```python
from build123d import *

# Parameters (mm, degrees)
F0_R     = 11.2
F1_DEPTH = 7


with BuildPart() as f1:
    # F0 (on Top) → F1 (new body)
    with BuildSketch(Plane.XY):
        with BuildLine():
            ThreePointArc((-0.9650827881, 13.1646730006), (-8.6022624346, 10.012046794), (-12.8691579618, 2.9367964443))
            ThreePointArc((-12.8691579618, 2.9367964443), (-13.1863620091, 0.599880793), (-13.0826534178, -1.7561832335))
            ThreePointArc((-13.0826534178, -1.7561832335), (-8.9594650145, -9.693708612), (-0.722399634, -13.1802177057))
            ThreePointArc((-0.722399634, -13.1802177057), (0, -13.1604354113), (0.722399634, -13.1802177057))
            ThreePointArc((0.722399634, -13.1802177057), (8.0432942537, -10.4663946777), (12.5501283831, -4.0907551342))
            ThreePointArc((12.5501283831, -4.0907551342), (13.0365197552, -2.0710269606), (13.2, 0))
            ThreePointArc((13.2, 0), (9.6689992451, 8.9861256167), (0.9650827881, 13.1646730006))
            ThreePointArc((0.9650827881, 13.1646730006), (0, 13.1293460011), (-0.9650827881, 13.1646730006))
        make_face()
        Circle(F0_R, mode=Mode.SUBTRACT)
        with BuildLine():
            ThreePointArc((-13.0826534178, -1.7561832335), (-13.1863620091, 0.599880793), (-12.8691579618, 2.9367964443))
            ThreePointArc((-12.8691579618, 2.9367964443), (-18.9175577348, 12.787783411), (-12.6283316175, 22.4867894878))
            ThreePointArc((-12.6283316175, 22.4867894878), (-13.0313646183, 24.2261255691), (-13.1959884441, 26.0039401262))
            ThreePointArc((-13.1959884441, 26.0039401262), (-24.637001113, 12.0769373767), (-13.0826534178, -1.7561832335))
        make_face()
        with BuildLine():
            ThreePointArc((-12.6283316175, 22.4867894878), (-8.2414011401, 16.0182205898), (-0.9650827881, 13.1646730006))
            ThreePointArc((-0.9650827881, 13.1646730006), (0, 13.2), (0.9650827881, 13.1646730006))
            ThreePointArc((0.9650827881, 13.1646730006), (9.6689992451, 17.3432203845), (13.2, 26.3293460011))
            ThreePointArc((13.2, 26.3293460011), (-0.1627153004, 39.5283430741), (-13.1959884441, 26.0039401262))
            ThreePointArc((-13.1959884441, 26.0039401262), (-13.0313646183, 24.2261255691), (-12.6283316175, 22.4867894878))
        make_face()
        with Locations((0, 26.3293460011)):
            Circle(F0_R, mode=Mode.SUBTRACT)
        with BuildLine():
            ThreePointArc((0.9650827881, 13.1646730006), (0, 13.2), (-0.9650827881, 13.1646730006))
            ThreePointArc((-0.9650827881, 13.1646730006), (0, 13.1293460011), (0.9650827881, 13.1646730006))
        make_face()
        with BuildLine():
            ThreePointArc((0.722399634, -13.1802177057), (0, -13.1604354113), (-0.722399634, -13.1802177057))
            ThreePointArc((-0.722399634, -13.1802177057), (0, -13.2), (0.722399634, -13.1802177057))
        make_face()
        with BuildLine():
            ThreePointArc((0.722399634, -13.1802177057), (0, -13.2), (-0.722399634, -13.1802177057))
            ThreePointArc((-0.722399634, -13.1802177057), (-10.4506279527, -34.4242047158), (12.566049408, -30.4020195408))
            ThreePointArc((12.566049408, -30.4020195408), (13.0405493018, -28.4059363053), (13.2, -26.3604354113))
            ThreePointArc((13.2, -26.3604354113), (13.1998442738, -26.2963171862), (13.199377099, -26.2322004739))
            ThreePointArc((13.199377099, -26.2322004739), (9.5416209523, -17.2391707181), (0.722399634, -13.1802177057))
        make_face()
        with Locations((0, -26.3604354113)):
            Circle(F0_R, mode=Mode.SUBTRACT)
        with BuildLine():
            ThreePointArc((13.2, -26.3604354113), (13.0405493018, -28.4059363053), (12.566049408, -30.4020195408))
            ThreePointArc((12.566049408, -30.4020195408), (21.9144963269, -15.3893362984), (13.2, 0))
            ThreePointArc((13.2, 0), (13.0365197552, -2.0710269606), (12.5501283831, -4.0907551342))
            ThreePointArc((12.5501283831, -4.0907551342), (18.3451878997, -15.001069441), (13.199377099, -26.2322004739))
            ThreePointArc((13.199377099, -26.2322004739), (13.1998442738, -26.2963171862), (13.2, -26.3604354113))
        make_face()
    extrude(amount=F1_DEPTH)


solid = f1.part
```
CAD build for the part. Positions are in the model's coordinates, mm. Coordinates: 2 decimals unless noted, no trailing zeros. Order: outer loops, then holes, each group sorted by start corner. A loop starts at its lowest first (then second) coordinate and runs counter-clockwise, first axis right, second up. Notation, with made-up numbers: (-30.75, -10) - (24.25, -10) arc R12 ccw to (24.25, -6) - close; hole circle Ø2 at (87.5, 51.5). An arc over 180 degrees is marked (long way). Use a Markdown table: item, result. Add a question column.
(1) Saw through at C-C (x = 16). Give the cut face in (y, z), then the cut area to 3 significant figures.
(2) Drill centre lines: line 1 along Y through (x, z) = (0, 1.5); line 2 along Y through (x, z) = (8, 3.25); line 3 along X through (y, z) = (18, 1.5). Where is each one in solid material? Low to high. Write a range as [from, to].
(3) Saw through at A-A (y = 33). Give the cut face in (x, z).
(4) Saw through at D-D (y = -7.5). Give the cut face in (x, z), then the cut area to 3 significant figures.
(5) Pull direction Y, two halves, no side cores. Call faces 1 (the face through (8, -10.5, 3.5)), 2 (the face through (21.907, -15.649, 3.451)), 3 (the face through (-12, 0, 7)): +Y half, -Y half, draft (parallel to the pull), parting line (faces both ways), or undercut.
(6) Saw through at B-B (x = 4.5). Give the cut face in (y, z).
(7) Flat gauge pins, fed straight in: pin 1 (5 mm diameter, centred on x = 14.5, y = -14.5, fed in from +Z); pin 2 (3 mm diameter, centred on y = 23.5, z = 1.5, fed in from +X); pin 3 (3 mm diameter, centred on y = -8, z = 5, fed in from +X); pin 4 (4 mm diameter, centred on y = 22, z = 1.5, fed in from +X). Where does each tip first touch, or does it go through?
Solved:
| question | item | result |
|---|---|---|
| 1 | outline | (-28.06, 0) - (-23.16, 0) - (-23.16, 7) - (-28.06, 7) - close; (-7.66, 0) - (-1.99, 0) - (-1.99, 7) - (-7.66, 7) - close |
| 1 | area | 74.0 mm² |
| 2 | line 1 | y = [-39.56, -37.56], [-15.16, -11.2], [11.2, 15.13], [37.53, 39.53] |
| 2 | line 2 | y = [-36.86, -34.2], [-18.52, -15.86], [-10.5, -7.84], [7.84, 10.5], [15.83, 18.49], [34.17, 36.83] |
| 2 | line 3 | x = [-23.36, -17.51], [-10.24, -7.49], [7.49, 10.24] |
| 3 | outline | (-11.39, 0) - (-9, 0) - (-9, 7) - (-11.39, 7) - close; (9, 0) - (11.39, 0) - (11.39, 7) - (9, 7) - close |
| 4 | outline | (-10.86, 0) - (-8.32, 0) - (-8.32, 7) - (-10.86, 7) - close; (8.32, 0) - (10.86, 0) - (10.86, 7) - (8.32, 7) - close; (15.89, 0) - (20.2, 0) - (20.2, 7) - (15.89, 7) - close |
| 4 | area | 65.8 mm² |
| 5 | face 1 | undercut |
| 5 | face 2 | parting line |
| 5 | face 3 | draft |
| 6 | outline | (-38.77, 0) - (-36.62, 0) - (-36.62, 7) - (-38.77, 7) - close; (-16.1, 0) - (-13.95, 0) - (-13.95, 7) - (-16.1, 7) - close; (-12.41, 0) - (-10.26, 0) - (-10.26, 7) - (-12.41, 7) - close; (10.26, 0) - (12.41, 0) - (12.41, 7) - (10.26, 7) - close; (13.92, 0) - (16.07, 0) - (16.07, 7) - (13.92, 7) - close; (36.59, 0) - (38.74, 0) - (38.74, 7) - (36.59, 7) - close |
| 7 | pin 1 | passes through |
| 7 | pin 2 | stops at x = 13.13 |
| 7 | pin 3 | stops at x = 21.01 |
| 7 | pin 4 | stops at x = 12.99 |
